```python
from build123d import *

# Parameters (mm, degrees)
SKETCH1_R           = 1.6
BOSS_EXTRUDE1_DEPTH = 27
CUT_EXTRUDE1_REACH  = 138.335
SKETCH2_R           = 2.1
CUT_EXTRUDE2_REACH  = 155.174
SKETCH3_R           = 1.7
SKETCH3_3_R         = 3
SKETCH3_3_R_2       = 1.7
CUT_EXTRUDE3_DEPTH  = 3
SKETCH4_R           = 3
CUT_EXTRUDE4_DEPTH  = 15


with BuildPart() as part:
    # Sketch1 → Boss-Extrude1 (new body)
    with BuildSketch(Plane.XY.offset(10)):
        with BuildLine():
            Line((-25.534872354, -37.053613776), (50.619597549, -89.534180987))
            ThreePointArc((50.619597549, -89.534180987), (54.361803385, -90.334528675), (57.573873786, -88.254320829))
            Line((57.573873786, -88.254320829), (58.227827632, -87.305369414))
            ThreePointArc((58.227827632, -87.305369414), (59.02817532, -83.563163578), (56.947967474, -80.351093178))
            Line((56.947967474, -80.351093178), (-21.854778729, -26.045511066))
            ThreePointArc((-21.854778729, -26.045511066), (-26.045511066, 21.854778729), (21.854778729, 26.045511066))
            Line((21.854778729, 26.045511066), (89.019290298, -42.129978983))
            ThreePointArc((89.019290298, -42.129978983), (92.543786433, -43.620813626), (96.090160837, -42.182797794))
            Line((96.090160837, -42.182797794), (96.911137653, -41.373995292))
            ThreePointArc((96.911137653, -41.373995292), (98.401972296, -37.849499157), (96.963956464, -34.303124754))
            Line((96.963956464, -34.303124754), (32.056602073, 31.581232775))
            ThreePointArc((32.056602073, 31.581232775), (-34.47199994, 28.925442436), (-25.534872354, -37.053613776))
        make_face()
        with Locations((90.17973297, -37.494440018)):
            Circle(SKETCH1_R, mode=Mode.SUBTRACT)
        with Locations((68.973861607, -16.273907044)):
            Circle(SKETCH1_R, mode=Mode.SUBTRACT)
        with Locations((47.767990244, 4.946625931)):
            Circle(SKETCH1_R, mode=Mode.SUBTRACT)
        with Locations((18.75, 32.475952642)):
            Circle(SKETCH1_R, mode=Mode.SUBTRACT)
        with Locations((-6.511806663, 36.930290738)):
            Circle(SKETCH1_R, mode=Mode.SUBTRACT)
        with Locations((-28.726666617, 24.104535363)):
            Circle(SKETCH1_R, mode=Mode.SUBTRACT)
        with Locations((-37.5, 0)):
            Circle(SKETCH1_R, mode=Mode.SUBTRACT)
        with Locations((-28.726666617, -24.104535363)):
            Circle(SKETCH1_R, mode=Mode.SUBTRACT)
        with Locations((3.423348889, -47.901259716)):
            Circle(SKETCH1_R, mode=Mode.SUBTRACT)
        with Locations((28.003855203, -65.100059364)):
            Circle(SKETCH1_R, mode=Mode.SUBTRACT)
        with Locations((52.584361518, -82.298859012)):
            Circle(SKETCH1_R, mode=Mode.SUBTRACT)
    extrude(amount=BOSS_EXTRUDE1_DEPTH)

    # Sketch2 → Cut-Extrude1 (cut, up to next)
    with BuildSketch(Plane.XY.offset(37), mode=Mode.PRIVATE) as cut_extrude1_sk1:
        with Locations((52.584361518, -82.298859012)):
            Circle(SKETCH2_R)
    cut_extrude1_tool1 = extrude(cut_extrude1_sk1.sketch, amount=-CUT_EXTRUDE1_REACH, mode=Mode.PRIVATE) & part.part
    # Sketch2 → Cut-Extrude1 (cut, up to next)
    with BuildSketch(Plane.XY.offset(37), mode=Mode.PRIVATE) as cut_extrude1_sk2:
        with Locations((28.003855203, -65.100059364)):
            Circle(SKETCH2_R)
    cut_extrude1_tool2 = extrude(cut_extrude1_sk2.sketch, amount=-CUT_EXTRUDE1_REACH, mode=Mode.PRIVATE) & part.part
    # Sketch2 → Cut-Extrude1 (cut, up to next)
    with BuildSketch(Plane.XY.offset(37), mode=Mode.PRIVATE) as cut_extrude1_sk3:
        with Locations((3.423348889, -47.901259716)):
            Circle(SKETCH2_R)
    cut_extrude1_tool3 = extrude(cut_extrude1_sk3.sketch, amount=-CUT_EXTRUDE1_REACH, mode=Mode.PRIVATE) & part.part
    # Sketch2 → Cut-Extrude1 (cut, up to next)
    with BuildSketch(Plane.XY.offset(37), mode=Mode.PRIVATE) as cut_extrude1_sk4:
        with Locations((-28.726666617, -24.104535363)):
            Circle(SKETCH2_R)
    cut_extrude1_tool4 = extrude(cut_extrude1_sk4.sketch, amount=-CUT_EXTRUDE1_REACH, mode=Mode.PRIVATE) & part.part
    # Sketch2 → Cut-Extrude1 (cut, up to next)
    with BuildSketch(Plane.XY.offset(37), mode=Mode.PRIVATE) as cut_extrude1_sk5:
        with Locations((-37.5, 0)):
            Circle(SKETCH2_R)
    cut_extrude1_tool5 = extrude(cut_extrude1_sk5.sketch, amount=-CUT_EXTRUDE1_REACH, mode=Mode.PRIVATE) & part.part
    # Sketch2 → Cut-Extrude1 (cut, up to next)
    with BuildSketch(Plane.XY.offset(37), mode=Mode.PRIVATE) as cut_extrude1_sk6:
        with Locations((-28.726666617, 24.104535363)):
            Circle(SKETCH2_R)
    cut_extrude1_tool6 = extrude(cut_extrude1_sk6.sketch, amount=-CUT_EXTRUDE1_REACH, mode=Mode.PRIVATE) & part.part
    # Sketch2 → Cut-Extrude1 (cut, up to next)
    with BuildSketch(Plane.XY.offset(37), mode=Mode.PRIVATE) as cut_extrude1_sk7:
        with Locations((-6.511806663, 36.930290738)):
            Circle(SKETCH2_R)
    cut_extrude1_tool7 = extrude(cut_extrude1_sk7.sketch, amount=-CUT_EXTRUDE1_REACH, mode=Mode.PRIVATE) & part.part
    # Sketch2 → Cut-Extrude1 (cut, up to next)
    with BuildSketch(Plane.XY.offset(37), mode=Mode.PRIVATE) as cut_extrude1_sk8:
        with Locations((18.75, 32.475952642)):
            Circle(SKETCH2_R)
    cut_extrude1_tool8 = extrude(cut_extrude1_sk8.sketch, amount=-CUT_EXTRUDE1_REACH, mode=Mode.PRIVATE) & part.part
    # Sketch2 → Cut-Extrude1 (cut, up to next)
    with BuildSketch(Plane.XY.offset(37), mode=Mode.PRIVATE) as cut_extrude1_sk9:
        with Locations((47.767990244, 4.946625931)):
            Circle(SKETCH2_R)
    cut_extrude1_tool9 = extrude(cut_extrude1_sk9.sketch, amount=-CUT_EXTRUDE1_REACH, mode=Mode.PRIVATE) & part.part
    # Sketch2 → Cut-Extrude1 (cut, up to next)
    with BuildSketch(Plane.XY.offset(37), mode=Mode.PRIVATE) as cut_extrude1_sk10:
        with Locations((68.973861607, -16.273907044)):
            Circle(SKETCH2_R)
    cut_extrude1_tool10 = extrude(cut_extrude1_sk10.sketch, amount=-CUT_EXTRUDE1_REACH, mode=Mode.PRIVATE) & part.part
    # Sketch2 → Cut-Extrude1 (cut, up to next)
    with BuildSketch(Plane.XY.offset(37), mode=Mode.PRIVATE) as cut_extrude1_sk11:
        with Locations((90.17973297, -37.494440018)):
            Circle(SKETCH2_R)
    cut_extrude1_tool11 = extrude(cut_extrude1_sk11.sketch, amount=-CUT_EXTRUDE1_REACH, mode=Mode.PRIVATE) & part.part
    add(cut_extrude1_tool1.solids().sort_by_distance((52.584362, -82.298859, 37))[0], mode=Mode.SUBTRACT)
    add(cut_extrude1_tool2.solids().sort_by_distance((28.003855, -65.100059, 37))[0], mode=Mode.SUBTRACT)
    add(cut_extrude1_tool3.solids().sort_by_distance((3.423349, -47.90126, 37))[0], mode=Mode.SUBTRACT)
    add(cut_extrude1_tool4.solids().sort_by_distance((-28.726667, -24.104535, 37))[0], mode=Mode.SUBTRACT)
    add(cut_extrude1_tool5.solids().sort_by_distance((-37.5, 0, 37))[0], mode=Mode.SUBTRACT)
    add(cut_extrude1_tool6.solids().sort_by_distance((-28.726667, 24.104535, 37))[0], mode=Mode.SUBTRACT)
    add(cut_extrude1_tool7.solids().sort_by_distance((-6.511807, 36.930291, 37))[0], mode=Mode.SUBTRACT)
    add(cut_extrude1_tool8.solids().sort_by_distance((18.75, 32.475953, 37))[0], mode=Mode.SUBTRACT)
    add(cut_extrude1_tool9.solids().sort_by_distance((47.76799, 4.946626, 37))[0], mode=Mode.SUBTRACT)
    add(cut_extrude1_tool10.solids().sort_by_distance((68.973862, -16.273907, 37))[0], mode=Mode.SUBTRACT)
    add(cut_extrude1_tool11.solids().sort_by_distance((90.179733, -37.49444, 37))[0], mode=Mode.SUBTRACT)

    # Sketch3 → Cut-Extrude2 (cut, up to next)
    with BuildSketch(Plane(origin=(-25.534872354, -37.053613776, 0), x_dir=(0.823413639467006, -0.567441607867893, 0), z_dir=(-0.5674416078678929, -0.8234136394670059, 0)), mode=Mode.PRIVATE) as cut_extrude2_sk1:
        with Locations((15, 23.5)):
            Circle(SKETCH3_R)
    cut_extrude2_tool1 = extrude(cut_extrude2_sk1.sketch, amount=-CUT_EXTRUDE2_REACH, mode=Mode.PRIVATE) & part.part
    add(cut_extrude2_tool1.solids().sort_by_distance((-13.183668, -45.565238, 23.5))[0], mode=Mode.SUBTRACT)

    # Sketch3<3> → Cut-Extrude3 (cut)
    with BuildSketch(Plane(origin=(-25.534872354, -37.053613776, 0), x_dir=(0.823413639467006, -0.567441607867893, 0), z_dir=(-0.5674416078678929, -0.8234136394670059, 0))):
        with Locations((15, 23.5)):
            Circle(SKETCH3_3_R)
        with Locations((15, 23.5)):
            Circle(SKETCH3_3_R_2, mode=Mode.SUBTRACT)
    extrude(amount=-CUT_EXTRUDE3_DEPTH, mode=Mode.SUBTRACT)

    # Sketch4 → Cut-Extrude4 (cut)
    with BuildSketch(Plane.XY.offset(37)):
        with Locations((18.75, 32.475952642)):
            Circle(SKETCH4_R)
        with Locations((-28.726666617, 24.104535363)):
            Circle(SKETCH4_R)
        with Locations((-28.726666617, -24.104535363)):
            Circle(SKETCH4_R)
    extrude(amount=-CUT_EXTRUDE4_DEPTH, mode=Mode.SUBTRACT)


solid = part.part
```
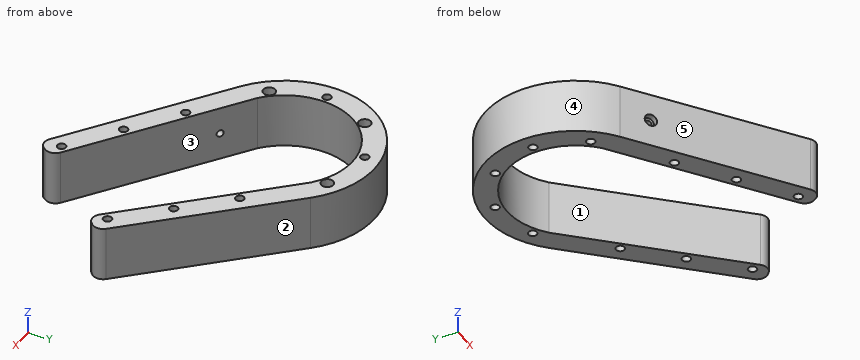
CAD build for the part. Positions are in the model's coordinates, mm. Face numbers are marked on the shaded views. A direction names the side the tool comes from. Coordinates: 2 decimals unless noted, no trailing zeros. Loops run counter-clockwise (first coordinate to the right, second up) from the corner with the lowest first, then second, coordinate; pieces in that order, holes last. Notation, with made-up numbers: (81.5, -21.5) - (134.5, -21.5) arc R12 ccw to (134.5, -10.5) - close; hole circle Ø6 at (56, 85.25). An arc over 180 degrees is marked (long way). Use CSV: the item, a comma, the result in double quotes. Start each with the question number.
Q1. Cut at C-C, the plane y = 0. List the corners of the cut face in (x, z).
Q2. Cut at D-D, the plane x = -29. List the corners of the cut face in (y, z), then the cut area to 3 significant figures.
Q3. Cut at B-B, the plane x = 39.5. List the corners of the cut face in (y, z), then the cut area to 3 significant figures.
Q4. Cut at A-A, the plane x = 18.75. List the corners of the cut face in (y, z), then the cut area to 3 significant figures.
Q5. Two-plate mould, pull along Y, no slides. Class the marked faces 3, 4 and 5: +Y half, -Y half, draft (parallel to the pull), parting line (faces both ways), or undercut.
Q6. Probe probe 1 along X at (y, z) = (25, 28); probe 2 along X at (y, z) = (-16, 21); probe 3 along Y at (x, z) = (4, 33). List the from-to ranges inside material, lowest first. Write a range as from..to.
Q7. 3-axis set-ups, long thin cutter, end or side, ignore diameter. For the marked faces 1 and 2: which of +Z, -Z, +X, -X, +Y, -Y reach the whole face in a straight line?
Q8. Drop flat-ended pins along their axis: P1, Ø3, axis at y = 4.5, z = 26.5, coming from the +X side; P2, Ø1.8, axis at x = -30, y = -25.5, coming from the +Z side; P3, Ø12, axis at x = 70.5, z = 13.5, coming from the -Y side. Give the stop position or say it passes through.
Here are the results:
1,outline,"(-45, 10) - (-39.6, 10) - (-39.6, 37) - (-45, 37) - close; (-35.4, 10) - (-34, 10) - (-34, 37) - (-35.4, 37) - close; (47.51, 10) - (63.17, 10) - (63.17, 37) - (47.51, 37) - close"
2,outline,"(-34.41, 10) - (-26.19, 10) - (-26.19, 22) - (-27.09, 22) - (-27.09, 37) - (-34.41, 37) - close; (-22.02, 10) - (-17.75, 10) - (-17.75, 37) - (-21.12, 37) - (-21.12, 22) - (-22.02, 22) - close; (17.75, 10) - (22.02, 10) - (22.02, 22) - (21.12, 22) - (21.12, 37) - (17.75, 37) - close; (26.19, 10) - (34.41, 10) - (34.41, 37) - (27.09, 37) - (27.09, 22) - (26.19, 22) - close"
2,area,"621 mm2"
3,outline,"(-81.87, 10) - (-68.33, 10) - (-68.33, 37) - (-81.87, 37) - close; (8.13, 10) - (24.03, 10) - (24.03, 37) - (8.13, 37) - close"
3,area,"795 mm2"
4,outline,"(-67.57, 10) - (-54.03, 10) - (-54.03, 37) - (-67.57, 37) - close; (28.36, 10) - (30.38, 10) - (30.38, 22) - (29.48, 22) - (29.48, 37) - (28.36, 37) - close; (34.58, 10) - (40.91, 10) - (40.91, 37) - (35.48, 37) - (35.48, 22) - (34.58, 22) - close"
4,area,"564 mm2"
5,face 3,"undercut"
5,face 4,"parting line"
5,face 5,"-Y half"
6,probe 1,"-37.42..-31.59, -25.86..-23.04, 22.88..38.54"
6,probe 2,"-42.06..-30, 63.28..66.89, 71.06..78.93"
6,probe 3,"-57.41..-49.92, -45.88..-43.86, 33.76..44.82"
7,face 1,"+Z, -Z"
7,face 2,"+Z, -Z, +X, +Y"
8,P1,"x = 60.21"
8,P2,"z = 22"
8,P3,"y = -29.42"
